Verification items for the finished model (mm, model axes). Face numbers are marked on the shaded views. A direction names the side the tool comes from. Round coordinates to 2 decimals unless told otherwise and drop trailing zeros. Order: outer loops, then holes, each group sorted by start corner. A loop starts at its lowest first (then second) coordinate and runs counter-clockwise, first axis right, second up. Notation, with made-up numbers: (30.25, -27) -> (44.25, -27) arc R23 cw to (44.25, -3) -> close; hole circle Ø10 at (61.5, -15). An arc over 180 degrees is marked (long way). Put each result on its own line as item: value.
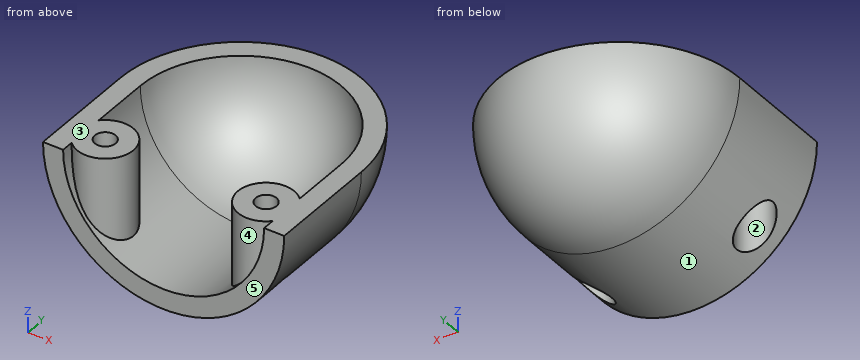
```python
from build123d import *

# Parameters (mm, degrees)
ROTATION1_ANGLE                 = 180
AUFSATZ_LINEAR_AUSTRAGEN1_REACH = 35.945
SKIZZE2_R                       = 3.5
SKIZZE4_R                       = 1.3
SCHNITT_LINEAR_AUSTRAGEN1_DEPTH = 34.944808145
SCHNITT_LINEAR_START            = -2
SKIZZE5_R                       = 2.25
SCHNITT_LINEAR_AUSTRAGEN2_DEPTH = 32.944808233


with BuildPart() as part:
    # Skizze1 → Rotation1 (revolve)
    with BuildSketch(Plane.XY):
        with BuildLine():
            Line((0, 26.5), (0, 24))
            ThreePointArc((0, 24), (-8.838834765, 20.338834765), (-12.5, 11.5))
            Line((-12.5, 11.5), (-12.5, 3.158312395))
            Line((-12.5, 3.158312395), (-12.5, -0.158312395))
            Line((-12.5, -0.158312395), (-12.5, -2.5))
            Line((-12.5, -2.5), (-15, -2.5))
            Line((-15, -2.5), (-15, 11.5))
            ThreePointArc((-15, 11.5), (-10.606601718, 22.106601718), (0, 26.5))
        make_face()
    revolve(axis=Axis((0, 26.5, 0), (0, -1, 0)), revolution_arc=ROTATION1_ANGLE)

    # Skizze2 → Aufsatz-Linear austragen1 (add, up to next)
    with BuildSketch(Plane.XY, mode=Mode.PRIVATE) as aufsatz_linear_austragen1_sk1:
        with Locations((-10, 1.5)):
            Circle(SKIZZE2_R)
        with BuildLine():
            ThreePointArc((-12.5, -0.158312395), (-7, 1.5), (-12.5, 3.158312395))
            Line((-12.5, 3.158312395), (-12.5, -0.158312395))
        make_face(mode=Mode.SUBTRACT)
    aufsatz_linear_austragen1_tool1 = extrude(aufsatz_linear_austragen1_sk1.sketch, amount=-AUFSATZ_LINEAR_AUSTRAGEN1_REACH, mode=Mode.PRIVATE) - part.part
    # Skizze2 → Aufsatz-Linear austragen1 (add, up to next)
    with BuildSketch(Plane.XY, mode=Mode.PRIVATE) as aufsatz_linear_austragen1_sk2:
        with BuildLine():
            Line((-12.5, 3.158312395), (-12.5, -0.158312395))
            ThreePointArc((-12.5, -0.158312395), (-7, 1.5), (-12.5, 3.158312395))
        make_face()
    aufsatz_linear_austragen1_tool2 = extrude(aufsatz_linear_austragen1_sk2.sketch, amount=-AUFSATZ_LINEAR_AUSTRAGEN1_REACH, mode=Mode.PRIVATE) - part.part
    aufsatz_linear_austragen1_1 = aufsatz_linear_austragen1_tool1.solids().sort_by_distance((-13.401005, 1.5, 0))[0]
    add(aufsatz_linear_austragen1_1)
    aufsatz_linear_austragen1_2 = aufsatz_linear_austragen1_tool2.solids().sort_by_distance((-9.888016, 1.5, 0))[0]
    add(aufsatz_linear_austragen1_2)
    aufsatz_linear_austragen1 = aufsatz_linear_austragen1_1 + aufsatz_linear_austragen1_2  # Aufsatz-Linear austragen1 as one shape, for the pattern or mirror that repeats it

    # Skizze4 → Schnitt-Linear austragen1 (cut, through all)
    with BuildSketch(Plane.XY):
        with Locations((-10, 1.5)):
            Circle(SKIZZE4_R)
    schnitt_linear_austragen1 = extrude(amount=-SCHNITT_LINEAR_AUSTRAGEN1_DEPTH, mode=Mode.SUBTRACT)

    # Skizze5 → Schnitt-Linear austragen2 (cut, through all)
    with BuildSketch(Plane.XY.offset(SCHNITT_LINEAR_START)):
        with Locations((-10, 1.5)):
            Circle(SKIZZE5_R)
    schnitt_linear_austragen2 = extrude(amount=-SCHNITT_LINEAR_AUSTRAGEN2_DEPTH, mode=Mode.SUBTRACT)

    # Spiegeln1: Aufsatz-Linear austragen1, Schnitt-Linear austragen1, Schnitt-Linear austragen2 across plane
    add(aufsatz_linear_austragen1.mirror(Plane(origin=(0, 0, 0), x_dir=(0, 0, 1), z_dir=(1, 0, 0))))
    add(schnitt_linear_austragen1.mirror(Plane(origin=(0, 0, 0), x_dir=(0, 0, 1), z_dir=(1, 0, 0))), mode=Mode.SUBTRACT)
    add(schnitt_linear_austragen2.mirror(Plane(origin=(0, 0, 0), x_dir=(0, 0, 1), z_dir=(1, 0, 0))), mode=Mode.SUBTRACT)


solid = part.part
```
Item 1: Tool access check on the marked faces 1 and 2. Record the directions out of +Z, -Z, +X, -X, +Y, -Y that give a thin tool (end or side, any length) a straight path to the whole face; none if there is none.
Geometry check:
face 1: -Z, +Y, -Y
face 2: -Z
Item 2: Sectioned sample at D-D, the plane x = -0.5. Record the boundary of the cut face in (y, z).
Geometry check:
outline: (-2.5, -14.99) -> (11.5, -14.99) arc R14.99 ccw to (26.49, 0) -> (23.99, 0) arc R12.49 cw to (11.5, -12.49) -> (-2.5, -12.49) -> close
Item 3: Material ranges on line 1 along Y through (x, z) = (-10, -1.15); line 2 along X through (y, z) = (1.5, -4.5); line 3 along Y through (x, z) = (10, -1.55), recorded low to high.
Geometry check:
line 1: -2 to 0.2, 2.8 to 5, 18.91 to 22.62
line 2: -14.31 to -12.25, -7.75 to -6.5, 6.5 to 7.75, 12.25 to 14.31
line 3: -2 to 0.2, 2.8 to 5, 18.84 to 22.57
Item 4: Depth check by flat-ended pin: pin 1 Ø1 at (y, z) = (6.5, -3) entering from +X; pin 2 Ø4 at (x, z) = (10.5, -10.5) entering from +Y; pin 3 Ø3 at (x, y) = (4, 1.5) entering from +Z (3 decimals). Enter the tip coordinate at first touch or a pass-through.
Geometry check:
pin 1: x = 14.79
pin 2: y = 19.24
pin 3: z = -11.225
Item 5: Sectioned sample at B-B, the plane x = -10. Record the boundary of the cut face in (y, z).
Geometry check:
outline: (-2.5, -11.18) -> (-0.75, -11.18) -> (-0.75, -2) -> (0.2, -2) -> (0.2, 0) -> (-2, 0) -> (-2, -7.5) -> (-2.5, -7.5) -> close; (2.8, -2) -> (3.75, -2) -> (3.75, -11.18) -> (11.5, -11.18) arc R11.18 ccw to (22.68, 0) -> (19, 0) arc R7.5 cw to (11.5, -7.5) -> (5, -7.5) -> (5, 0) -> (2.8, 0) -> close
Item 6: Release check for a two-part mould opening along Y. For the marked faces 3, 4 and 5 record: pulls with the +Y half, pulls with the -Y half, needs draft (parallel to the pull), parting line crosses it, or undercut.
Geometry check:
face 3: needs draft
face 4: undercut
face 5: pulls with the -Y half
Item 7: Sectioned sample at C-C, the plane z = -5.25. Record the boundary of the cut face in (x, y), then the cut area to 3 significant figures.
Geometry check:
outline: (-14.05, -2.5) -> (-11.34, -2.5) -> (-11.34, -1.73) arc R3.5 ccw (long way) to (-11.34, 4.73) -> (-11.34, 11.5) arc R11.34 cw to (11.34, 11.5) -> (11.34, 4.73) arc R3.5 ccw (long way) to (11.34, -1.73) -> (11.34, -2.5) -> (14.05, -2.5) -> (14.05, 11.5) arc R14.05 ccw to (-14.05, 11.5) -> close; hole circle Ø4.5 at (-10, 1.5); hole circle Ø4.5 at (10, 1.5)
area: 209 mm2
Item 8: Sectioned sample at A-A, the plane y = 1.5. Record the boundary of the cut face in (x, z), then the cut area to 3 significant figures.
Geometry check:
outline: (-15, 0) arc R15 ccw to (-12.25, -8.66) -> (-12.25, -2) -> (-11.3, -2) -> (-11.3, 0) -> close; (-8.7, -2) -> (-7.75, -2) -> (-7.75, -12.84) arc R15 ccw to (7.75, -12.84) -> (7.75, -2) -> (8.7, -2) -> (8.7, 0) -> (6.5, 0) -> (6.5, -10.68) arc R12.5 cw to (-6.5, -10.68) -> (-6.5, 0) -> (-8.7, 0) -> close; (11.3, -2) -> (12.25, -2) -> (12.25, -8.66) arc R15 ccw to (15, 0) -> (11.3, 0) -> close
area: 107 mm2
